```python
from build123d import *

# Parameters (mm, degrees)
F0_W        = 152.4
F0_H        = 101.6
F1_DEPTH    = 127
F2_T        = -2.54
F3_T1_DEPTH = 117.475
F3_T3_DEPTH = 168.275


# Not quite as in the source:
# - a fillet or chamfer that OpenCascade refuses, or shapes differently, is made with other operations: its cross-section is extruded or revolved along the edge and cut away or added


with BuildPart() as f1:
    # F0 (on Top) → F1 (new body)
    with BuildSketch(Plane.XY):
        with Locations((76.2, 50.8)):
            Rectangle(F0_W, F0_H)
    extrude(amount=F1_DEPTH)

    # F2
    f2_openings = [f1.faces().sort_by_distance(p)[0] for p in [
        (76.2, 50.8, 127),
    ]]
    offset(amount=F2_T, openings=f2_openings)

    # F3: fillet of radius 3.175 on 4 edges, made by hand

    # F3_s2 → F3_t1 (cut)
    with BuildSketch(Plane.XZ.offset(-109.5375)):
        with BuildLine():
            ThreePointArc((0, 123.825), (0.9299359697, 126.0700640303), (3.175, 127))
            Line((3.175, 127), (0, 127))
            Line((0, 127), (0, 123.825))
        make_face()
        with BuildLine():
            ThreePointArc((152.4, 123.825), (151.4700640303, 126.0700640303), (149.225, 127))
            Line((149.225, 127), (152.4, 127))
            Line((152.4, 127), (152.4, 123.825))
        make_face()
    extrude(amount=F3_T1_DEPTH, mode=Mode.SUBTRACT)

    # F3_s4 → F3_t3 (cut)
    with BuildSketch(Plane.YZ.offset(-7.9375)):
        with BuildLine():
            ThreePointArc((0, 123.825), (0.9299359697, 126.0700640303), (3.175, 127))
            Line((3.175, 127), (0, 127))
            Line((0, 127), (0, 123.825))
        make_face()
        with BuildLine():
            ThreePointArc((101.6, 123.825), (100.6700640303, 126.0700640303), (98.425, 127))
            Line((98.425, 127), (101.6, 127))
            Line((101.6, 127), (101.6, 123.825))
        make_face()
    extrude(amount=F3_T3_DEPTH, mode=Mode.SUBTRACT)


solid = f1.part
```
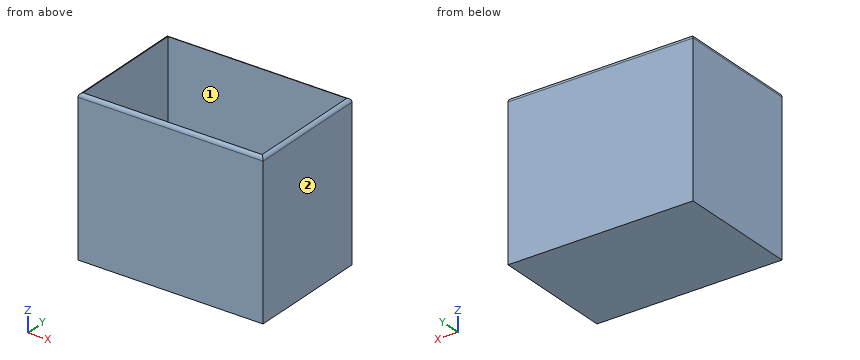
Input: part model. Units: mm. Frame: model coordinates. Face numbers are marked on the shaded views. A direction names the side the tool comes from. Coordinates: 2 decimals unless noted, no trailing zeros. Write each loop counter-clockwise with the first axis right and the second up, starting at its lowest first coordinate (ties: lowest second). Pieces come first, ordered by that corner, then holes. Notation, with made-up numbers: M 60.25,-29.75 L 66.25,-29.75 A31 ccw 66.25,1.25 Z; hole C 71.5,-1.75 d10. An arc over 180 degrees is marked long. Use one line per item in the form item = value.
Q1. First-contact query: pin 1 (2 mm diameter, centred on x = 52, y = 25, fed in from +Z). Flat tip, straight axial feed; report the tip coordinate or a pass-through.
Answer below:
pin_1 = 2.54
Q2. Section A-A (z = 13). Return loops of the section in (x, y).
Answer below:
outline = M 0,0 L 152.4,0 L 152.4,101.6 L 0,101.6 Z; hole M 2.54,2.54 L 149.86,2.54 L 149.86,99.06 L 2.54,99.06 Z
Q3. Material intervals for probe 1 along Y at (x, z) = (72.5, 32.5); probe 2 along X at (y, z) = (85, 75.5); probe 3 along Z at (x, y) = (146, 76), sorted ascending. Write a range as from..to.
Answer below:
probe_1 = 0..2.54, 99.06..101.6
probe_2 = 0..2.54, 149.86..152.4
probe_3 = 0..2.54
Q4. Section B-B (y = 17). Return loops of the section in (x, z) (3 decimals), plus the area to 3 significant figures.
Answer below:
outline = M 0,0 L 152.4,0 L 152.4,123.825 A3.175 ccw 149.86,126.936 L 149.86,2.54 L 2.54,2.54 L 2.54,126.936 A3.175 ccw 0,123.825 Z
area = 1,020 mm²
Q5. Set-up query: the marked faces 1 and 2. Return all of +Z, -Z, +X, -X, +Y, -Y with unobstructed straight access to the full face (end or side cutting, diameter ignored); none if empty.
Answer below:
face_1 = +Z
face_2 = +Z, -Z, +X, +Y, -Y
Q6. Section C-C (x = 132). Return loops of the section in (y, z) (3 decimals), plus the area to 3 significant figures.
Answer below:
outline = M 0,0 L 101.6,0 L 101.6,123.825 A3.175 ccw 99.06,126.936 L 99.06,2.54 L 2.54,2.54 L 2.54,126.936 A3.175 ccw 0,123.825 Z
area = 886 mm²
